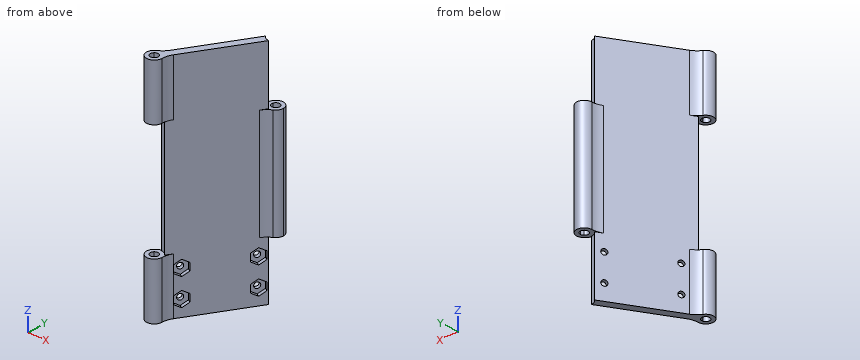
from build123d import *

# Parameters (mm, degrees)
SKETCH2_R               = 1.5875
BOSS_EXTRUDE1_DEPTH     = 10
BOSS_EXTRUDE2_DEPTH     = 120
SKETCH4_R               = 4.0875
CUT_EXTRUDE1_DEPTH      = 30.5
CUT_EXTRUDE1_DEPTH_BACK = 30.5
SKETCH5_R               = 4.0875
CUT_EXTRUDE2_DEPTH      = 31
SKETCH6_R               = 4.0875
CUT_EXTRUDE3_DEPTH      = 31
FILLET1_R               = 10
SKETCH7_R               = 1.5
CUT_EXTRUDE4_DEPTH      = 4
SKETCH8_R               = 1.5
CUT_EXTRUDE5_DEPTH      = 2


with BuildPart() as part:
    # Sketch2 → Boss-Extrude1 (new body)
    with BuildSketch(Plane.XY):
        with BuildLine():
            Line((0, -27.7495), (0, 0))
            Line((0, 0), (38.1, 0))
            ThreePointArc((38.1, 0), (-26.940768363, 26.940768363), (0, -38.1))
            Line((0, -38.1), (0, -30.9245))
            ThreePointArc((0, -30.9245), (-1.5875, -29.337), (0, -27.7495))
        make_face()
        with Locations((-25.406587271, 14.6685)):
            Circle(SKETCH2_R, mode=Mode.SUBTRACT)
        with Locations((25.406587271, 14.6685)):
            Circle(SKETCH2_R, mode=Mode.SUBTRACT)
        with BuildLine():
            Line((38.1, 0), (0, 0))
            Line((0, 0), (0, -27.7495))
            ThreePointArc((0, -27.7495), (1.122532015, -28.214467985), (1.5875, -29.337))
            ThreePointArc((1.5875, -29.337), (1.122532015, -30.459532015), (0, -30.9245))
            Line((0, -30.9245), (0, -38.1))
            ThreePointArc((0, -38.1), (26.940768363, -26.940768363), (38.1, 0))
        make_face()
    extrude(amount=BOSS_EXTRUDE1_DEPTH)


with BuildPart() as body_2:
    # Sketch3 → Boss-Extrude2 (new body)
    with BuildSketch(Plane.XY.offset(10)):
        with BuildLine():
            ThreePointArc((29.494087271, 14.6685), (24.324372064, 18.610132466), (21.892146477, 12.581309985))
            Line((21.892146477, 12.581309985), (23.37551462, 15.150578976))
            ThreePointArc((23.37551462, 15.150578976), (25.649272347, 16.741845172), (27.494087271, 14.6685))
            ThreePointArc((27.494087271, 14.6685), (27.323499399, 13.841998855), (26.839616236, 13.150578976))
            Line((26.839616236, 13.150578976), (25.356248092, 10.581309985))
            ThreePointArc((25.356248092, 10.581309985), (28.279033516, 11.760457906), (29.494087271, 14.6685))
        make_face()
        with BuildLine():
            Line((24.362837271, 12.86067197), (23.362837271, 11.128621162))
            ThreePointArc((23.362837271, 11.128621162), (24.324372064, 10.726867534), (25.356248092, 10.581309985))
            Line((25.356248092, 10.581309985), (26.839616236, 13.150578976))
            ThreePointArc((26.839616236, 13.150578976), (25.649272347, 12.595154828), (24.362837271, 12.86067197))
        make_face()
        with BuildLine():
            ThreePointArc((21.892146477, 12.581309985), (22.534141026, 11.760457906), (23.362837271, 11.128621162))
            Line((23.362837271, 11.128621162), (24.362837271, 12.86067197))
            ThreePointArc((24.362837271, 12.86067197), (23.489675143, 13.841998855), (23.37551462, 15.150578976))
            Line((23.37551462, 15.150578976), (21.892146477, 12.581309985))
        make_face()
        with BuildLine():
            Line((23.362837271, 11.128621162), (2.04375, -25.797121162))
            ThreePointArc((2.04375, -25.797121162), (2.872446245, -26.428957906), (3.514440794, -27.249809985))
            Line((3.514440794, -27.249809985), (25.356248092, 10.581309985))
            ThreePointArc((25.356248092, 10.581309985), (24.324372064, 10.726867534), (23.362837271, 11.128621162))
        make_face()
        with BuildLine():
            ThreePointArc((0.050339179, -25.249809985), (1.082215206, -25.395367534), (2.04375, -25.797121162))
            Line((2.04375, -25.797121162), (23.362837271, 11.128621162))
            ThreePointArc((23.362837271, 11.128621162), (22.534141026, 11.760457906), (21.892146477, 12.581309985))
            Line((21.892146477, 12.581309985), (0.050339179, -25.249809985))
        make_face()
        with BuildLine():
            ThreePointArc((-1.433028965, -27.819078976), (-0.242685076, -27.263654828), (1.04375, -27.52917197))
            Line((1.04375, -27.52917197), (2.04375, -25.797121162))
            ThreePointArc((2.04375, -25.797121162), (1.082215206, -25.395367534), (0.050339179, -25.249809985))
            Line((0.050339179, -25.249809985), (-1.433028965, -27.819078976))
        make_face()
        with BuildLine():
            Line((2.04375, -25.797121162), (1.04375, -27.52917197))
            ThreePointArc((1.04375, -27.52917197), (1.80782803, -28.29325), (2.0875, -29.337))
            ThreePointArc((2.0875, -29.337), (2.073345172, -29.579685076), (2.03107265, -29.819078976))
            Line((2.03107265, -29.819078976), (3.514440794, -27.249809985))
            ThreePointArc((3.514440794, -27.249809985), (2.872446245, -26.428957906), (2.04375, -25.797121162))
        make_face()
        with BuildLine():
            ThreePointArc((2.03107265, -29.819078976), (-1.04375, -31.14482803), (-1.433028965, -27.819078976))
            Line((-1.433028965, -27.819078976), (0.050339179, -25.249809985))
            ThreePointArc((0.050339179, -25.249809985), (-2.908042094, -32.209446245), (4.0875, -29.337))
            ThreePointArc((4.0875, -29.337), (3.941632466, -28.254784794), (3.514440794, -27.249809985))
            Line((3.514440794, -27.249809985), (2.03107265, -29.819078976))
        make_face()
    extrude(amount=BOSS_EXTRUDE2_DEPTH)

    # Sketch4 → Cut-Extrude1 (cut, two sides)
    with BuildSketch(Plane.XY.offset(70)) as cut_extrude1_sk:
        with Locations((0, -29.337)):
            Circle(SKETCH4_R)
    extrude(amount=CUT_EXTRUDE1_DEPTH, mode=Mode.SUBTRACT)
    extrude(cut_extrude1_sk.sketch, amount=-CUT_EXTRUDE1_DEPTH_BACK, mode=Mode.SUBTRACT)

    # Sketch5 → Cut-Extrude2 (cut)
    with BuildSketch(Plane(origin=(0, 0, 10), x_dir=(-1, 0, 0), z_dir=(0, 0, -1))):
        with Locations((-25.406587271, 14.6685)):
            Circle(SKETCH5_R)
    extrude(amount=-CUT_EXTRUDE2_DEPTH, mode=Mode.SUBTRACT)

    # Sketch6 → Cut-Extrude3 (cut)
    with BuildSketch(Plane.XY.offset(130)):
        with Locations((25.406587271, 14.6685)):
            Circle(SKETCH6_R)
    extrude(amount=-CUT_EXTRUDE3_DEPTH, mode=Mode.SUBTRACT)

    # Fillet1
    fillet1_edges = [body_2.edges().sort_by_distance(p)[0] for p in [
        (0.050339179, -25.249809985, 115.25),
        (3.514440794, -27.249809985, 115.25),
        (0.050339179, -25.249809985, 24.75),
        (3.514440794, -27.249809985, 24.75),
        (21.892146477, 12.581309985, 70),
        (25.356248092, 10.581309985, 70),
    ]]
    fillet(fillet1_edges, radius=FILLET1_R)

    # Sketch7 → Cut-Extrude4 (cut)
    with BuildSketch(Plane(origin=(10.971242828, -6.33425, 0), x_dir=(0, 0, 1), z_dir=(-0.866025404, 0.5, 0))):
        with Locations((18.38424077, -14.582087011)):
            Circle(SKETCH7_R)
        with Locations((18.38424077, 17.647912989)):
            Circle(SKETCH7_R)
        with Locations((32.55424077, 17.647912989)):
            Circle(SKETCH7_R)
        with Locations((32.55424077, -14.582087011)):
            Circle(SKETCH7_R)
    extrude(amount=-CUT_EXTRUDE4_DEPTH, mode=Mode.SUBTRACT)

    # Sketch8 → Cut-Extrude5 (cut)
    with BuildSketch(Plane(origin=(14.435344443, -8.33425, 0), x_dir=(0, 0, -1), z_dir=(0.866025404, -0.5, 0))):
        with Locations((-18.38424077, -14.582087011)):
            Circle(SKETCH8_R)
        Polygon((-34.516051881, 14.208627429), (-30.556637659, 14.22929195), (-28.594826548, 17.66857751), (-30.592429659, 21.08719855), (-34.55184388, 21.066534029), (-36.513654991, 17.627248469), align=None)
        with Locations((-18.38424077, 17.647912989)):
            Circle(SKETCH8_R)
        Polygon((-34.516051881, -18.021372571), (-30.556637659, -18.00070805), (-28.594826548, -14.56142249), (-30.592429659, -11.14280145), (-34.55184388, -11.163465971), (-36.513654991, -14.602751531), align=None)
        with Locations((-32.55424077, 17.647912989)):
            Circle(SKETCH8_R)
        Polygon((-20.346051881, -18.021372571), (-16.386637659, -18.00070805), (-14.424826548, -14.56142249), (-16.422429659, -11.14280145), (-20.38184388, -11.163465971), (-22.343654991, -14.602751531), align=None)
        Polygon((-20.346051881, 14.208627429), (-16.386637659, 14.22929195), (-14.424826548, 17.66857751), (-16.422429659, 21.08719855), (-20.38184388, 21.066534029), (-22.343654991, 17.627248469), align=None)
    extrude(amount=-CUT_EXTRUDE5_DEPTH, mode=Mode.SUBTRACT)


solid = body_2.part
Geometry: final body of the model. Coordinates: model frame, mm. Give positions to 0.01 mm unless a question says otherwise; leave off trailing zeros. Loops run counter-clockwise (first coordinate to the right, second up) from the corner with the lowest first, then second, coordinate; pieces in that order, holes last. Notation, with made-up numbers: M 56.25,-37.75 L 99.25,-37.75 A11 ccw 99.25,-33.75 Z; hole C 69.25,61.5 d7. An arc over 180 degrees is marked long. Put each result on its own line as item: value. Start each with the question number.
1) Contact query for flat-ended pins moving along their axis: pin 1 (2 mm diameter, centred on y = 2.5, z = 108.5, fed in from +X); pin 2 (6 mm diameter, centred on y = -20.5, z = 102, fed in from -X); pin 3 (5 mm diameter, centred on x = 24, y = 14.5, fed in from +Z); pin 4 (4 mm diameter, centred on x = 0, y = -29.337, fed in from -Z). Output: stop coordinate, or through.
2) Cut plane A-A (z = 106). Output: boundary loops of the cut face in (x, y) (1 decimal).
3) Ray query, line 1 along X through (y, z) = (-11.5, 52.5); line 2 along Y through (x, z) = (0, 115.5); line 3 along Z through (x, y) = (19.5, 8). Return the intervals inside material, ascending.
4) Cut plane C-C (y = -12.5). Output: boundary loops of the cut face in (x, z), then the cut area to 3 significant figures.
5) Cut plane B-B (x = 13.5). Output: boundary loops of the cut face in (y, z), then the cut area to 3 significant figures.
Verdict:
1. pin 1: x = 21.27
1. pin 2: x = 0.85
1. pin 3: z = 99
1. pin 4: through
2. outline: M -1.9,-25.7 A4.1 ccw long 4.1,-29.2 A10 cw 5.4,-23.9 L 25.4,10.6 A4.1 cw 21.9,12.6 L 2,-21.9 A10 cw Z; hole C 0,-29.3 d4.2
3. line 1: 7.99 to 12.61
3. line 2: -33.42 to -31.42, -27.25 to -24.37
3. line 3: 10 to 17.24, 19.53 to 31.41, 33.7 to 130
4. outline: M 7.41,10 L 12.03,10 L 12.03,130 L 7.41,130 Z
4. area: 554 mm2
5. outline: M -9.95,10 L -1.95,10 L -1.95,130 L -9.95,130 Z
5. area: 960 mm2
